Geometry check sheet. Reference: drawing and pictorial views, mm from the part's lowest x, y, z. A direction names the side the tool comes from. Round coordinates to 2 decimals unless told otherwise and drop trailing zeros. Loops run counter-clockwise (first coordinate to the right, second up) from the corner with the lowest first, then second, coordinate; pieces in that order, holes last. Notation, with made-up numbers: (-11, -21.75) - (-4, -21.75) arc R17 cw to (-4, -9.75) - close; hole circle Ø1 at (88.5, 75). An arc over 180 degrees is marked (long way). Answer as CSV lines item,"result". Start each with the question number.
1) Cross-section at C-C on z = 4.6. Record the boundary of the cut face in (x, y).
2) Draft check along Y on the marked faces 1, 2 and 3. Enter one of: released by +Y, released by -Y, zero draft, split by the parting line, or undercut.
3) Access from +Z, -Z, +X, -X, +Y, -Y to the whole of each face (thin tool, end or side, straight path). Record for the marked faces 4 and 5.
4) Thickness scan on line 1 along Y through (x, z) = (9.75, 1.7); line 2 along X through (y, z) = (14, 1). Record the ranges inside material, lowest first.
5) Cross-section at B-B on y = 5.25. Record the boundary of the cut face in (x, z).
6) Cross-section at A-A on x = 9.25. Record the boundary of the cut face in (y, z).
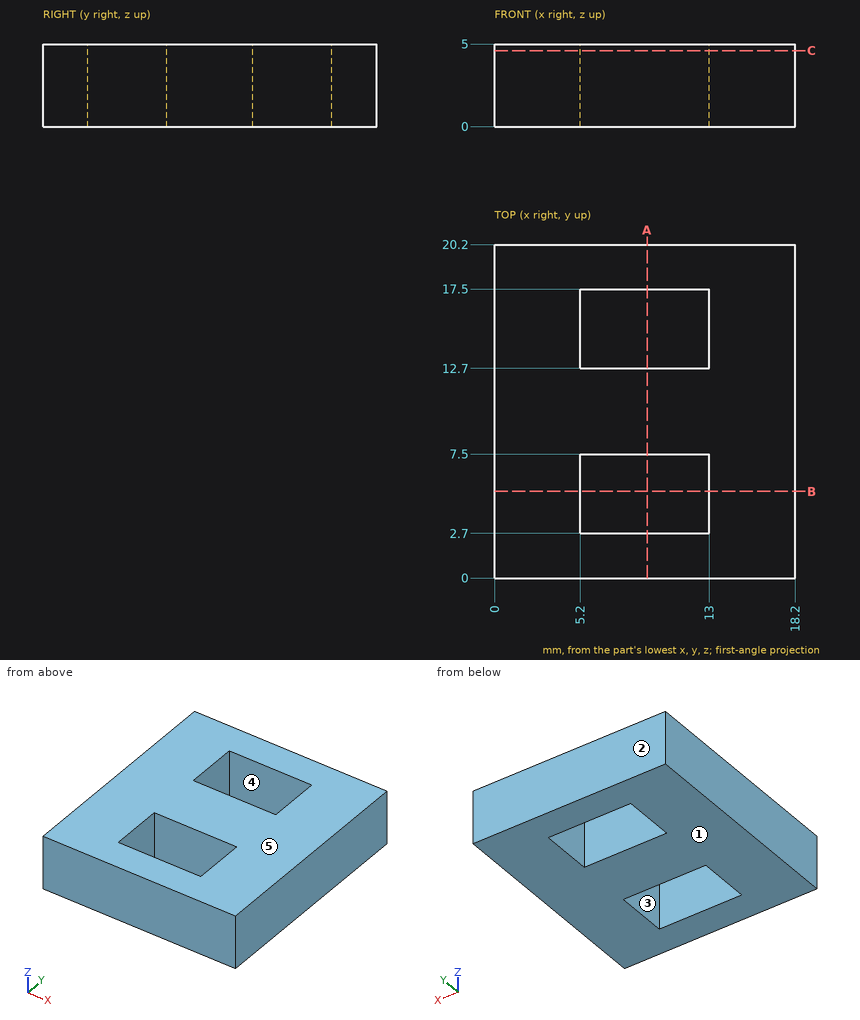
Answer block:
1,outline,"(0, 0) - (18.2, 0) - (18.2, 20.2) - (0, 20.2) - close; hole (5.2, 2.7) - (13, 2.7) - (13, 7.5) - (5.2, 7.5) - close; hole (5.2, 12.7) - (13, 12.7) - (13, 17.5) - (5.2, 17.5) - close"
2,face 1,"zero draft"
2,face 2,"released by +Y"
2,face 3,"undercut"
3,face 4,"+Z, -Z"
3,face 5,"+Z, +X, -X, +Y, -Y"
4,line 1,"y = 0 to 2.7, 7.5 to 12.7, 17.5 to 20.2"
4,line 2,"x = 0 to 5.2, 13 to 18.2"
5,outline,"(0, 0) - (5.2, 0) - (5.2, 5) - (0, 5) - close; (13, 0) - (18.2, 0) - (18.2, 5) - (13, 5) - close"
6,outline,"(0, 0) - (2.7, 0) - (2.7, 5) - (0, 5) - close; (7.5, 0) - (12.7, 0) - (12.7, 5) - (7.5, 5) - close; (17.5, 0) - (20.2, 0) - (20.2, 5) - (17.5, 5) - close"
